from build123d import *

# Parameters (mm, degrees)
SKETCH4_W               = 80
SKETCH4_H               = 40
SKETCH4_R               = 4.75
SKETCH4_R_2             = 4.5
BOSS_EXTRUDE2_DEPTH     = 25
CUT_EXTRUDE3_DEPTH      = 52.23475383
CUT_EXTRUDE3_DEPTH_BACK = 52.23475383
SKETCH5_W               = 34
SKETCH5_H               = 60
CUT_EXTRUDE4_DEPTH      = 52.23475383
CUT_EXTRUDE4_DEPTH_BACK = 52.23475383
SKETCH6_R               = 4.75
FILLET1_R               = 20
FILLET3_R               = 15


with BuildPart() as part:
    # Sketch4 → Boss-Extrude2 (new, symmetric)
    with BuildSketch(Plane(origin=(0, 0, 0), x_dir=(0, 0, -1), z_dir=(1, 0, 0))):
        Rectangle(SKETCH4_W, SKETCH4_H)
        with Locations((-25, 10)):
            Circle(SKETCH4_R, mode=Mode.SUBTRACT)
        with Locations((-25, -11)):
            Circle(SKETCH4_R_2, mode=Mode.SUBTRACT)
    extrude(amount=BOSS_EXTRUDE2_DEPTH, both=True)

    # Sketch5 → Cut-Extrude3 (cut, two sides: drawn at the far end of the back side and taken through both)
    with BuildSketch(Plane(origin=(0, 0, 0), x_dir=(1, 0, 0), z_dir=(0, 1, 0)).offset(-CUT_EXTRUDE3_DEPTH_BACK)):
        with Locations((0, -10)):
            Rectangle(SKETCH5_W, SKETCH5_H)
    extrude(amount=CUT_EXTRUDE3_DEPTH + CUT_EXTRUDE3_DEPTH_BACK, mode=Mode.SUBTRACT)

    # Sketch6 → Cut-Extrude4 (cut, two sides: drawn at the far end of the back side and taken through both)
    with BuildSketch(Plane(origin=(0, 0, 0), x_dir=(1, 0, 0), z_dir=(0, 1, 0)).offset(-CUT_EXTRUDE4_DEPTH_BACK)):
        with Locations(Location((0, 30, 0), (0, 0, 270))):
            Circle(SKETCH6_R)
    extrude(amount=CUT_EXTRUDE4_DEPTH + CUT_EXTRUDE4_DEPTH_BACK, mode=Mode.SUBTRACT)

    # Fillet1
    fillet1_edges = [part.edges().sort_by_distance(p)[0] for p in [
        (25, 0, -40),
        (-25, 0, -40),
    ]]
    fillet(fillet1_edges, radius=FILLET1_R)

    # Fillet3
    fillet3_edges = [part.edges().sort_by_distance(p)[0] for p in [
        (-21, -20, 40),
        (-21, 20, 40),
        (21, -20, 40),
        (21, 20, 40),
    ]]
    fillet(fillet3_edges, radius=FILLET3_R)


solid = part.part
Here's how the part is built. I have some questions about the finished solid (model axes, mm). A direction names the side the tool comes from. Give positions to 0.01 mm unless a question says otherwise; leave off trailing zeros. Loops run counter-clockwise (first coordinate to the right, second up) from the corner with the lowest first, then second, coordinate; pieces in that order, holes last. Notation, with made-up numbers: (-33.5, -39) -> (-12.5, -39) arc R27 cw to (-12.5, -7) -> close; hole circle Ø9 at (84, 87). An arc over 180 degrees is marked (long way). Answer as a JSON object with one key per item and string values. Group by question number.
Item 1: I need wall thicknesses on L1, parallel to X at y = 15, z = -8; L2, parallel to Y at x = 19, z = 28; L3, parallel to Y at x = -21, z = 24. Which ranges of each line are inside material? Lowest first, please.
Item 2: Imagine slicing it at B-B on y = 10. Write out the boundary of the cut face in (x, z), then the cut area to 3 significant figures.
Item 3: Imagine slicing it at C-C on y = -1. Write out the boundary of the cut face in (x, z), then the cut area to 3 significant figures.
Item 4: Will these pins go through, and if not, where does the flat tip stop? pin 1 (1 mm diameter, centred on x = 19, y = -9.5, fed in from +Z); pin 2 (5.5 mm diameter, centred on y = -11, z = 25, fed in from -X); pin 3 (1 mm diameter, centred on x = -19.5, y = -9, fed in from +Z); pin 4 (10 mm diameter, centred on x = 18, y = -3, fed in from -Z).
Item 5: Thinking about a two-plate mould opening in Y: for faces 1 (the cylindrical face through (21.06, -15.72, 35.49)), 2 (the cylindrical face through (20.944, 8.181, 20.612)), 3 (the flat face through (21, 0, 40)), which applies, pulls with the +Y half, pulls with the -Y half, needs draft (parallel to the pull), parting line crosses it, or undercut?
Item 6: Imagine slicing it at A-A on z = 34. Write out the boundary of the cut face in (x, y), then the cut area to 3 significant figures.
Item 7: Imagine slicing it at D-D on z = 9.5. Write out the boundary of the cut face in (x, y).
Item 8: On a 3-axis mill with a long thin cutter (end or side, diameter ignored), from which of +Z, -Z, +X, -X, +Y, -Y can I reach the whole of each face in a straight line? I mean faces 4 (the flat face through (0, 20, -21)), 5 (the flat face through (-17, 0, 10)). Say none if no direction works.
Answer list:
{
 "1": {"L1": "x = -25 to -17, 17 to 25", "L2": "y = -19.7 to -14.35, -7.65 to 6.32, 13.68 to 19.7", "L3": "y = -20 to -15.39, -6.61 to 5.36, 14.64 to 20"},
 "2": {"outline": "(-25, -20) arc R20 ccw to (-5, -40) -> (5, -40) arc R20 ccw to (25, -20) -> (25, 20.25) -> (17, 20.25) -> (17, -20) -> (-17, -20) -> (-17, 20.25) -> (-25, 20.25) -> close; (-25, 29.75) -> (-17, 29.75) -> (-17, 39.14) -> (-25, 39.14) -> close; (17, 29.75) -> (25, 29.75) -> (25, 39.14) -> (17, 39.14) -> close; hole circle Ø9.5 at (0, -30)", "area": "1,550 mm2"},
 "3": {"outline": "(-25, -20) arc R20 ccw to (-5, -40) -> (5, -40) arc R20 ccw to (25, -20) -> (25, 40) -> (17, 40) -> (17, -20) -> (-17, -20) -> (-17, 40) -> (-25, 40) -> close; hole circle Ø9.5 at (0, -30)", "area": "1,720 mm2"},
 "4": {"pin 1": "stops at z = 39.46", "pin 2": "passes through", "pin 3": "stops at z = 39.59", "pin 4": "stops at z = -38.33"},
 "5": {"face 1": "pulls with the -Y half", "face 2": "undercut", "face 3": "needs draft"},
 "6": {"outline": "(-25, -17) -> (-17, -17) -> (-17, 17) -> (-25, 17) -> close; (17, -17) -> (25, -17) -> (25, 17) -> (17, 17) -> close", "area": "544 mm2"},
 "7": {"outline": "(-25, -20) -> (-17, -20) -> (-17, 20) -> (-25, 20) -> close; (17, -20) -> (25, -20) -> (25, 20) -> (17, 20) -> close"},
 "8": {"face 4": "+Z, -Z, +X, -X, +Y", "face 5": "+Z, +Y, -Y"}
}
